Can you work these out from the drawing? Everything is in mm from the part's minimum corner. Coordinates: 2 decimals unless noted, no trailing zeros. Order: outer loops, then holes, each group sorted by start corner. A loop starts at its lowest first (then second) coordinate and runs counter-clockwise, first axis right, second up. Notation, with made-up numbers: M 71.5,2.25 L 120.5,2.25 A25 ccw 120.5,36.25 Z; hole C 21,-21.75 d7. An arc over 180 degrees is marked long. One line per question, with ' | ' between items. Start each with the question number.
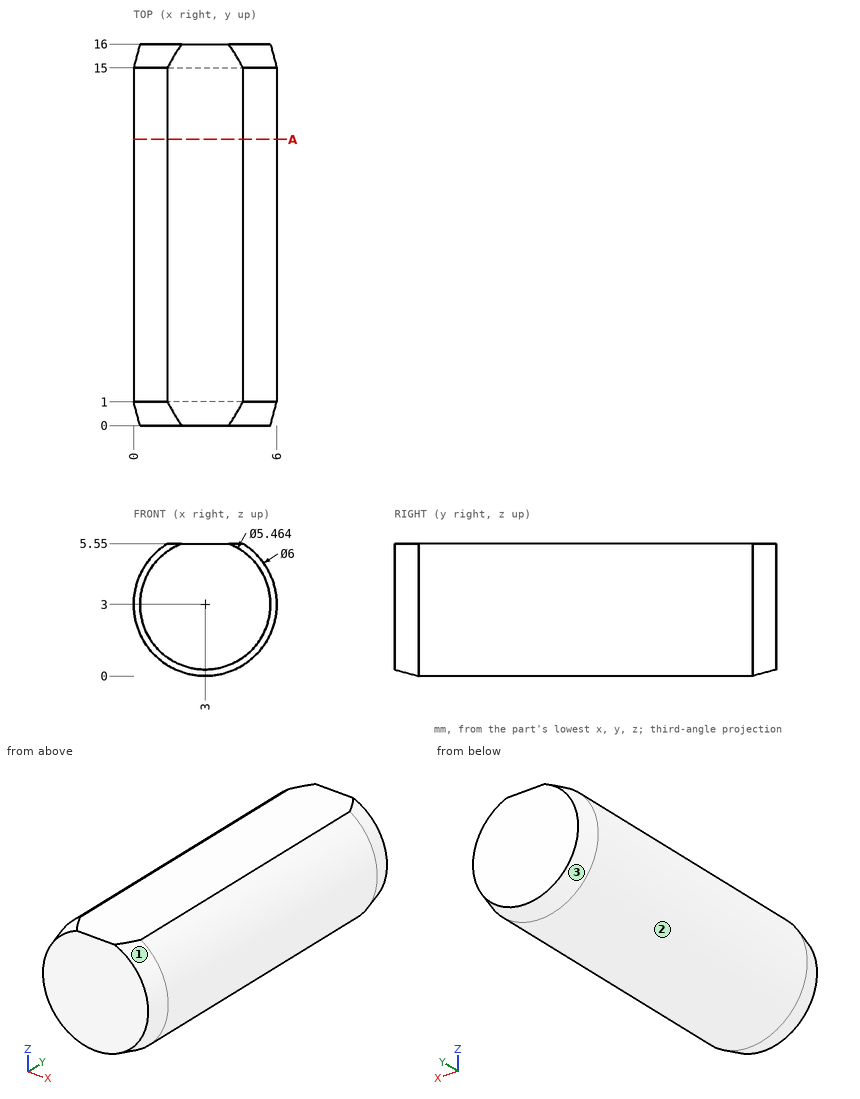
(1) Imagine slicing it at A-A, the plane y = 12. Write out the boundary of the cut face in (x, z), plus the area to 3 significant figures.
(2) For P1, Ø2, axis at y = 11.5, z = 1, coming from the -X side, with a flat end and sliding along its axis, tell me the tip position at first contact or that it passes through.
(3) We'd pull the mould along Y, two halves only. Please class the marked faces 1, 2 and 3: +Y half, -Y half, draft (parallel to the pull), parting line (faces both ways), or undercut.
(4) If I drill on line 1 along X through (y, z) = (9.5, 2.85); line 2 along Z through (x, y) = (1.25, 2.5); line 3 along X through (y, z) = (13.25, 4.1), over which ranges is the centre line in solid material (lowest first)? Write a range as from..to.
Answers:
1) outline: M 1.42,5.55 A3 ccw long 4.58,5.55 Z | area: 27.3 mm²
2) P1: x = 0.17
3) face 1: -Y half | face 2: draft | face 3: +Y half
4) line 1: 0..6 | line 2: 0.56..5.44 | line 3: 0.21..5.79
